from build123d import *

# Parameters (mm, degrees)
BOSS_EXTRUDE1_DEPTH = 2.5
SKETCH2_W           = 15
SKETCH2_H           = 5
BOSS_EXTRUDE2_DEPTH = 12.5
BOSS_EXTRUDE3_DEPTH = 1.5
SKETCH6_R           = 2.15
CUT_EXTRUDE1_DEPTH  = 5


with BuildPart() as part:
    # Sketch1 → Boss-Extrude1 (new, symmetric)
    with BuildSketch(Plane.XY):
        Polygon((-12.5, 45), (-7.5, 50), (7.5, 50), (12.5, 45), (12.5, -50), (-12.5, -50), align=None)
        with BuildLine():
            Line((9.5, 23), (9.5, -37))
            ThreePointArc((9.5, -37), (7.4, -39.1), (5.3, -37))
            Line((5.3, -37), (5.3, 23))
            ThreePointArc((5.3, 23), (7.4, 25.1), (9.5, 23))
        make_face(mode=Mode.SUBTRACT)
        with BuildLine():
            Line((-9.5, 23), (-9.5, -37))
            ThreePointArc((-9.5, -37), (-7.4, -39.1), (-5.3, -37))
            Line((-5.3, -37), (-5.3, 23))
            ThreePointArc((-5.3, 23), (-7.4, 25.1), (-9.5, 23))
        make_face(mode=Mode.SUBTRACT)
    extrude(amount=BOSS_EXTRUDE1_DEPTH, both=True)

    # Sketch2 → Boss-Extrude2 (add, symmetric)
    with BuildSketch(Plane(origin=(0, 0, 0), x_dir=(0, 0, -1), z_dir=(1, 0, 0))):
        with Locations((10, -47.5)):
            Rectangle(SKETCH2_W, SKETCH2_H)
        with Locations((-10, -47.5)):
            Rectangle(SKETCH2_W, SKETCH2_H)
    extrude(amount=BOSS_EXTRUDE2_DEPTH, both=True)

    # Sketch5 → Boss-Extrude3 (add, symmetric)
    with BuildSketch(Plane(origin=(0, 0, 0), x_dir=(0, 0, -1), z_dir=(1, 0, 0))):
        Polygon((-14.5, -45), (-2.5, -33), (-2.5, -45), align=None)
        Polygon((2.5, -33), (2.5, -45), (14.5, -45), align=None)
    extrude(amount=BOSS_EXTRUDE3_DEPTH, both=True)

    # Sketch6 → Cut-Extrude1 (cut)
    with BuildSketch(Plane(origin=(0, -45, 0), x_dir=(1, 0, 0), z_dir=(0, 1, 0))):
        with Locations(Location((-7, 10, 0), (0, 0, 270))):
            Circle(SKETCH6_R)
        with Locations(Location((7, 10, 0), (0, 0, 270))):
            Circle(SKETCH6_R)
        with Locations(Location((7, -10, 0), (0, 0, 270))):
            Circle(SKETCH6_R)
        with Locations(Location((-7, -10, 0), (0, 0, 270))):
            Circle(SKETCH6_R)
    extrude(amount=-CUT_EXTRUDE1_DEPTH, mode=Mode.SUBTRACT)


solid = part.part
The model under review builds one solid part; all positions refer to its coordinate system, in mm. A direction names the side the tool comes from. Round coordinates to 2 decimals unless told otherwise and drop trailing zeros. Order: outer loops, then holes, each group sorted by start corner. A loop starts at its lowest first (then second) coordinate and runs counter-clockwise, first axis right, second up. Notation, with made-up numbers: (2.5, 76) -> (34.5, 76) arc R24 ccw to (34.5, 94) -> close; hole circle Ø9 at (15, -39). An arc over 180 degrees is marked (long way). Use CSV: the item, a comma, the result in double quotes. Start each with the question number.
(1) Mouldability with a two-part tool opening along X and no side actions: class faces 5 (the face through (0, -50, 0)), 6 (the face through (-7.4, 25.1, 0)), 7 (the face through (-10, 47.5, 0)), 8 (the face through (1.5, -42, 6)) as pulls with the +X half, pulls with the -X half, needs draft (parallel to the pull), parting line crosses it, or undercut.
(2) Consider section D-D on z = -1. Write out the cut boundary in (x, y).
(3) Tool access review of faces 1 (the face through (1.5, -42, -6)), 2 (the face through (-3, -45, -10)), 3 (the face through (7.4, -39.1, 0)), 4 (the face through (0, 50, 0)): name each direction out of +Z, -Z, +X, -X, +Y, -Y from which nothing blocks a thin tool from reaching the whole face with its end or side.
(4) Insertion check: pin 1 (6 mm diameter, centred on x = -4, z = -12, fed in from +Y); pin 2 (12.5 mm diameter, centred on x = 2.5, y = 0.5, fed in from +Z); pin 3 (2.5 mm diameter, centred on x = 7, z = -10, fed in from +Y); pin 4 (1 mm diameter, centred on x = 7.5, z = -7, fed in from +Y). Each pin has a flat end and moves straight along its axis. Give the tip position at first contact, or say it passes through.
(5) Wall thickness on probe 1 along X at (y, z) = (0, 1); probe 2 along X at (y, z) = (-47, 10); probe 3 along Y at (x, z) = (-2, 16): over which ranges is each line inside the solid? List them lowest first. Write a range as from..to.
(6) Consider section B-B on z = -10. Write out the cut boundary in (x, y), and give its area (3 significant figures).
(7) Consider section A-A on y = -28. Write out the cut boundary in (x, z), and give its area (3 significant figures).
(8) Consider section C-C on x = 10.5. Write out the cut boundary in (y, z).
Responses:
1,face 5,"needs draft"
1,face 6,"undercut"
1,face 7,"pulls with the -X half"
1,face 8,"pulls with the +X half"
2,outline,"(-12.5, -50) -> (12.5, -50) -> (12.5, 45) -> (7.5, 50) -> (-7.5, 50) -> (-12.5, 45) -> close; hole (-9.5, -37) arc R2.1 ccw to (-5.3, -37) -> (-5.3, 23) arc R2.1 ccw to (-9.5, 23) -> close; hole (5.3, -37) arc R2.1 ccw to (9.5, -37) -> (9.5, 23) arc R2.1 ccw to (5.3, 23) -> close"
3,face 1,"-Z, +X, +Y"
3,face 2,"-Z, +Y"
3,face 3,"+Z, -Z"
3,face 4,"+Z, -Z, +X, -X, +Y"
4,pin 1,"y = -40.84"
4,pin 2,"z = 2.5"
4,pin 3,"through"
4,pin 4,"y = -45"
5,probe 1,"-12.5..-9.5, -5.3..5.3, 9.5..12.5"
5,probe 2,"-12.5..-9.15, -4.85..4.85, 9.15..12.5"
5,probe 3,"-50..-45"
6,outline,"(-12.5, -50) -> (-9.15, -50) -> (-9.15, -45) -> (-12.5, -45) -> close; (-4.85, -50) -> (4.85, -50) -> (4.85, -45) -> (1.5, -45) -> (1.5, -40.5) -> (-1.5, -40.5) -> (-1.5, -45) -> (-4.85, -45) -> close; (9.15, -50) -> (12.5, -50) -> (12.5, -45) -> (9.15, -45) -> close"
6,area,"95.5 mm²"
7,outline,"(-12.5, -2.5) -> (-9.5, -2.5) -> (-9.5, 2.5) -> (-12.5, 2.5) -> close; (-5.3, -2.5) -> (5.3, -2.5) -> (5.3, 2.5) -> (-5.3, 2.5) -> close; (9.5, -2.5) -> (12.5, -2.5) -> (12.5, 2.5) -> (9.5, 2.5) -> close"
7,area,"83.0 mm²"
8,outline,"(-50, -17.5) -> (-45, -17.5) -> (-45, -2.5) -> (47, -2.5) -> (47, 2.5) -> (-45, 2.5) -> (-45, 17.5) -> (-50, 17.5) -> close"
